from build123d import *

# Parameters (mm, degrees)
CROQUIS1_R              = 23.5
CROQUIS1_R_2            = 1.5
SALIENTE_EXTRUIR1_DEPTH = 1.8
CROQUIS2_W              = 21
CROQUIS2_H              = 16
CORTAR_EXTRUIR1_DEPTH   = 0.2


with BuildPart() as part:
    # Croquis1 → Saliente-Extruir1 (new body)
    with BuildSketch(Plane.XY):
        Circle(CROQUIS1_R)
        with Locations((0, -20.2)):
            Circle(CROQUIS1_R_2, mode=Mode.SUBTRACT)
        with Locations((-12.5, 13.5)):
            Circle(CROQUIS1_R_2, mode=Mode.SUBTRACT)
        with Locations((12.5, 13.5)):
            Circle(CROQUIS1_R_2, mode=Mode.SUBTRACT)
    extrude(amount=SALIENTE_EXTRUIR1_DEPTH)

    # Croquis2 → Cortar-Extruir1 (cut)
    with BuildSketch(Plane.XY.offset(1.8)):
        with Locations((-5, -5)):
            Rectangle(CROQUIS2_W, CROQUIS2_H)
    extrude(amount=-CORTAR_EXTRUIR1_DEPTH, mode=Mode.SUBTRACT)


solid = part.part
Input: part model. Units: mm. Frame: model coordinates. Give positions to 0.01 mm unless a question says otherwise; leave off trailing zeros. Order: outer loops, then holes, each group sorted by start corner. A loop starts at its lowest first (then second) coordinate and runs counter-clockwise, first axis right, second up.
Q1. Section D-D on y = 0. Output: boundary loops of the cut face in (x, z), and give its area (3 significant figures).
Checked values:
outline: (-23.5, 0) - (23.5, 0) - (23.5, 1.8) - (5.5, 1.8) - (5.5, 1.6) - (-15.5, 1.6) - (-15.5, 1.8) - (-23.5, 1.8) - close
area: 80.4 mm2
Q2. Section A-A on x = 13. Output: boundary loops of the cut face in (y, z).
Checked values:
outline: (-19.58, 0) - (12.09, 0) - (12.09, 1.8) - (-19.58, 1.8) - close; (14.91, 0) - (19.58, 0) - (19.58, 1.8) - (14.91, 1.8) - close
Q3. Ray query, probe 1 along Y at (x, z) = (0, 0.65); probe 2 along Z at (x, y) = (-7, 2); probe 3 along Y at (x, z) = (-13, 0.25). Return the intervals inside material, ascending.
Checked values:
probe 1: y = -23.5 to -21.7, -18.7 to 23.5
probe 2: z = 0 to 1.6
probe 3: y = -19.58 to 12.09, 14.91 to 19.58
Q4. Section C-C on z = 0.5. Output: boundary loops of the cut face in (x, y).
Checked values:
outline: circle Ø47 at (0, 0); hole circle Ø3 at (-12.5, 13.5); hole circle Ø3 at (0, -20.2); hole circle Ø3 at (12.5, 13.5)
Q5. Contact query for flat-ended pins moving along their axis: pin 1 Ø1 at (y, z) = (2, 1) entering from +X; pin 2 Ø2.5 at (x, y) = (-12.5, 13.5) entering from +Z; pin 3 Ø5 at (x, y) = (-10, -7) entering from +Z. Output: stop coordinate, or through.
Checked values:
pin 1: stops at x = 23.45
pin 2: passes through
pin 3: stops at z = 1.6
Q6. Draft query along X for faces 1 (the flat face through (0, 0, 0)), 2 (the flat face through (-5, -5, 1.6)), 3 (the cylindrical face through (22.4, 7.1, 0.9)). Return one class per face: +X half, -X half, draft (parallel to the pull), parting line (faces both ways), or undercut.
Checked values:
face 1: draft
face 2: undercut
face 3: parting line
Q7. Section B-B on y = 13.5. Output: boundary loops of the cut face in (x, z).
Checked values:
outline: (-19.24, 0) - (-14, 0) - (-14, 1.8) - (-19.24, 1.8) - close; (-11, 0) - (11, 0) - (11, 1.8) - (-11, 1.8) - close; (14, 0) - (19.24, 0) - (19.24, 1.8) - (14, 1.8) - close
